Check sheet for the modelled part. Datum: model origin and axes. Units: mm. Coordinates: 2 decimals unless noted, no trailing zeros. Write each loop counter-clockwise with the first axis right and the second up, starting at its lowest first coordinate (ties: lowest second). Pieces come first, ordered by that corner, then holes. Notation, with made-up numbers: (12.25, -10) - (40.25, -10) arc R20 cw to (40.25, 18) - close; hole circle Ø11 at (56.5, 26). An arc over 180 degrees is marked (long way). Answer as CSV lines item,"result". Start each with the question number.
from build123d import *

# Parameters (mm, degrees)
F1_DEPTH      = 37.5
F2_R          = 14.5799335076
F3_DEPTH      = 37.501
F3_DEPTH_BACK = 37.501
F4_R          = 5


with BuildPart() as f1:
    # F0 (on Top) → F1 (new body, symmetric)
    with BuildSketch(Plane.XY):
        with BuildLine():
            ThreePointArc((13.6289698518, -43.9534703049), (37.0461490082, -27.2990698509), (46.0180005113, 0))
            ThreePointArc((46.0180005113, 0), (37.0461490082, 27.2990698509), (13.6289698518, 43.9534703049))
            ThreePointArc((13.6289698518, 43.9534703049), (-46.0180005113, 0), (13.6289698518, -43.9534703049))
        make_face()
        with BuildLine():
            ThreePointArc((13.6289698518, 43.9534703049), (37.0461490082, 27.2990698509), (46.0180005113, 0))
            ThreePointArc((46.0180005113, 0), (37.0461490082, -27.2990698509), (13.6289698518, -43.9534703049))
            Line((13.6289698518, -43.9534703049), (103.4320995684, -16.1075655557))
            ThreePointArc((103.4320995684, -16.1075655557), (81.5733594357, 0), (103.4320995684, 16.1075655557))
            Line((103.4320995684, 16.1075655557), (13.6289698518, 43.9534703049))
        make_face()
        with BuildLine():
            ThreePointArc((115.3016614259, 0), (112.0137598054, 10.0042511816), (103.4320995684, 16.1075655557))
            ThreePointArc((103.4320995684, 16.1075655557), (81.5733594357, 0), (103.4320995684, -16.1075655557))
            ThreePointArc((103.4320995684, -16.1075655557), (112.0137598054, -10.0042511816), (115.3016614259, 0))
        make_face()
    extrude(amount=F1_DEPTH, both=True)

    # F2 (on Top) → F3 (cut, two sides)
    with BuildSketch(Plane.XY) as f3_sk:
        Circle(F2_R)
    extrude(amount=-F3_DEPTH, mode=Mode.SUBTRACT)
    extrude(f3_sk.sketch, amount=F3_DEPTH_BACK, mode=Mode.SUBTRACT)

    # F4
    f4_edges = [f1.edges().sort_by_distance(p)[0] for p in [
        (58.530535, -30.030518, 37.5),
    ]]
    fillet(f4_edges, radius=F4_R)


solid = f1.part
(1) Go/stop test with flat-tipped pins: P1, Ø4, axis at y = 12.5, z = -13, coming from the +X side; P2, Ø1, axis at x = -10.5, z = 27.5, coming from the -Y side; P3, Ø2, axis at y = -7, z = 21.5, coming from the +X side. Record where each tip stops, or that it passes through.
(2) Cross-section at A-A on z = 11. Record the boundary of the cut face in (x, y).
(3) Material ranges on probe 1 along Y at (x, z) = (0, -16.5); probe 2 along X at (y, z) = (0, 8); probe 3 along Z at (x, y) = (53.5, 26.5), recorded low to high. Write a range as from..to.
Checked values:
1,P1,"x = 111.63"
1,P2,"y = -44.92"
1,P3,"x = 114.2"
2,outline,"(13.63, -43.95) - (103.43, -16.11) arc R16.86 ccw to (103.43, 16.11) - (13.63, 43.95) arc R46.02 ccw (long way) to start; hole circle Ø29.16 at (0, 0)"
3,probe 1,"-46.02..-14.58, 14.58..46.02"
3,probe 2,"-46.02..-14.58, 14.58..115.3"
3,probe 3,"-37.5..37.5"
